Input: part model. Units: mm. Frame: model coordinates. Face numbers are marked on the shaded views. A direction names the side the tool comes from. Give positions to 0.01 mm unless a question says otherwise; leave off trailing zeros. Order: outer loops, then holes, each group sorted by start corner. A loop starts at its lowest first (then second) coordinate and runs counter-clockwise, first axis right, second up. Notation, with made-up numbers: (79, 28) -> (113, 28) arc R20 ccw to (113, 54) -> close; hole circle Ø6 at (19.5, 71.5). An arc over 180 degrees is marked (long way). Use a Markdown table: item, result. Add a question column.
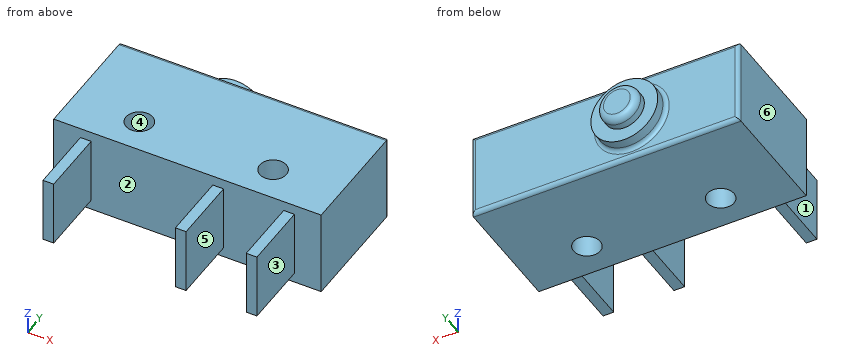
from build123d import *

# Parameters (mm, degrees)
SKETCH_W     = 20
SKETCH_H     = 9
SKETCH_R     = 1
PAD_DEPTH    = 3.25
SKETCH001_W  = 0.8
SKETCH001_H  = 5
PAD001_DEPTH = 2.5
FILLET_R     = 0.5
FILLET001_R  = 0.3


with BuildPart() as part:
    # Sketch → Pad (new body, symmetric)
    with BuildSketch(Plane.XY):
        with Locations((0, 4.5)):
            Rectangle(SKETCH_W, SKETCH_H)
        with Locations((-5, 2.5)):
            Circle(SKETCH_R, mode=Mode.SUBTRACT)
        with Locations((5, 2.5)):
            Circle(SKETCH_R, mode=Mode.SUBTRACT)
    extrude(amount=PAD_DEPTH, both=True)

    # Sketch001 → Pad001 (join, symmetric)
    with BuildSketch(Plane.XY):
        with Locations((-7.6, -2.5)):
            Rectangle(SKETCH001_W, SKETCH001_H)
        with Locations((7.6, -2.5)):
            Rectangle(SKETCH001_W, SKETCH001_H)
        with Locations((2.3, -2.5)):
            Rectangle(SKETCH001_W, SKETCH001_H)
    extrude(amount=PAD001_DEPTH, both=True)

    # Sketch002 → Revolution (revolve)
    with BuildSketch(Plane.XY):
        Polygon((-2, 9), (-4.5, 9), (-4.5, 10), (-3.5, 10), (-3.5, 11), (-2, 11), align=None)
    revolve(axis=Axis((-2, 0, 0), (0, -1, 0)))

    # Fillet
    fillet_edges = [part.edges().sort_by_distance(p)[0] for p in [
        (-0.5, 11, 0),
    ]]
    fillet(fillet_edges, radius=FILLET_R)

    # Fillet001
    fillet001_edges = [part.edges().sort_by_distance(p)[0] for p in [
        (10, 9, 0),
        (0, 9, -3.25),
        (0, 9, 3.25),
        (-10, 9, 0),
        (0.5, 9, 0),
    ]]
    fillet(fillet001_edges, radius=FILLET001_R)


solid = part.part
Q1. Draft query along X for the marked faces 1, 2, 3 and 4. Return one class per face: +X half, -X half, draft (parallel to the pull), parting line (faces both ways), or undercut.
Q2. Section query A-A (y = 2.5). Return loops of the section in (x, z), plus the area to 3 significant figures.
Q3. Section query D-D (x = 7.75). Return loops of the section in (y, z).
Q4. First-contact query: pin 1 (1.8 mm diameter, centred on x = 5, y = 2.5, fed in from -Z); pin 2 (1.5 mm diameter, centred on y = -3.5, z = 1, fed in from +X); pin 3 (1 mm diameter, centred on x = 1.5, z = -0.5, fed in from +Y); pin 4 (0.6 mm diameter, centred on x = -7.5, y = -2.5, fed in from -Z). Flat tips, straight axial feed; report the tip coordinate or a pass-through.
Q5. Ray query, line 1 (X direction, y = -2.5, z = 2); line 2 (Y direction, x = -5, z = 0.5); line 3 (Y direction, x = -2.25, z = -1). Return the intervals inside material, ascending.
Q6. Section query B-B (x = 5). Return loops of the section in (y, z).
Q7. Section query C-C (z = 0). Give the number of separate pieces and of enclosed holes in the cut face, plus the area to 3 significant figures.
Q8. Access query for the marked faces 5 and 6. Directions: +Z, -Z, +X, -X, +Y, -Y. A direction counts if a zero-diameter tool reaches every point of the face in a straight line with its end or side. Return the directions, or none.
Solution:
| question | item | result |
|---|---|---|
| 1 | face 1 | -X half |
| 1 | face 2 | undercut |
| 1 | face 3 | +X half |
| 1 | face 4 | undercut |
| 2 | outline | (-10, -3.25) -> (-6, -3.25) -> (-6, 3.25) -> (-10, 3.25) -> close; (-4, -3.25) -> (4, -3.25) -> (4, 3.25) -> (-4, 3.25) -> close; (6, -3.25) -> (10, -3.25) -> (10, 3.25) -> (6, 3.25) -> close |
| 2 | area | 104 mm² |
| 3 | outline | (-5, -2.5) -> (0, -2.5) -> (0, -3.25) -> (8.7, -3.25) arc R0.3 ccw to (9, -2.95) -> (9, 2.95) arc R0.3 ccw to (8.7, 3.25) -> (0, 3.25) -> (0, 2.5) -> (-5, 2.5) -> close |
| 4 | pin 1 | passes through |
| 4 | pin 2 | stops at x = 8 |
| 4 | pin 3 | stops at y = 9 |
| 4 | pin 4 | stops at z = -2.5 |
| 5 | line 1 | x = -8 to -7.2, 1.9 to 2.7, 7.2 to 8 |
| 5 | line 2 | y = 0 to 1.5, 3.5 to 9 |
| 5 | line 3 | y = 0 to 11 |
| 6 | outline | (0, -3.25) -> (1.5, -3.25) -> (1.5, 3.25) -> (0, 3.25) -> close; (3.5, -3.25) -> (8.7, -3.25) arc R0.3 ccw to (9, -2.95) -> (9, 2.95) arc R0.3 ccw to (8.7, 3.25) -> (3.5, 3.25) -> close |
| 7 | separate pieces | 1 |
| 7 | enclosed holes | 2 |
| 7 | area | 194 mm² |
| 8 | face 5 | +Z, -Z, -Y |
| 8 | face 6 | +Z, -Z, -X, +Y, -Y |
